Check sheet for the drawn part. Datum: minimum x, y, z corner. Units: mm. A direction names the side the tool comes from. Round coordinates to 2 decimals unless told otherwise and drop trailing zeros. Order: outer loops, then holes, each group sorted by start corner. A loop starts at its lowest first (then second) coordinate and runs counter-clockwise, first axis right, second up. Notation, with made-up numbers: (56.25, 75.5) -> (100.25, 75.5) arc R20 ccw to (100.25, 92.5) -> close; hole circle Ø6 at (-39, -23). An arc over 180 degrees is marked (long way). Use CSV: the item, a comma, the result in double quotes.
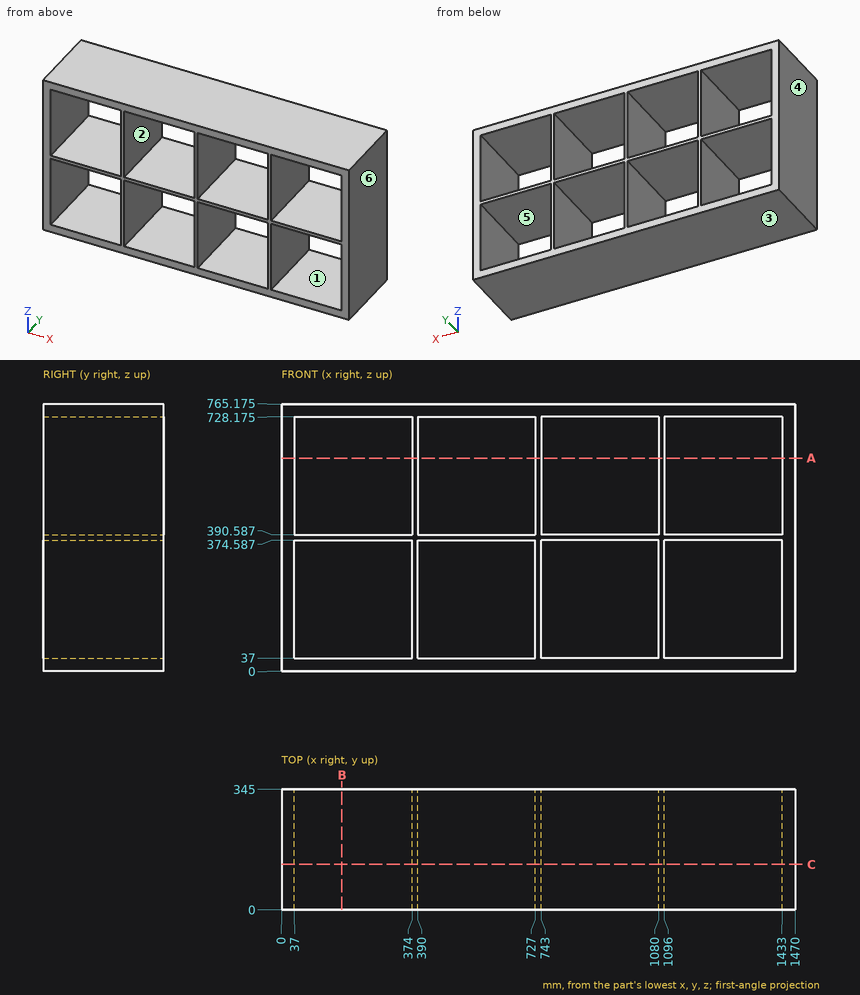
Q1. Sectioned sample at C-C, the plane y = 130. State how many separate pieces and enclosed holes the cut face has, then the cut area to 3 significant figures.
Result sheet:
separate pieces,"1"
enclosed holes,"8"
area,"215,000 mm^2"
Q2. Mould release check, pull along X, two halves, no side actions. Record for the marked faces 1, 2, 3 and 4: pulls with the +X half, pulls with the -X half, needs draft (parallel to the pull), parting line crosses it, or undercut.
Result sheet:
face 1,"undercut"
face 2,"undercut"
face 3,"needs draft"
face 4,"pulls with the -X half"
Q3. Sectioned sample at B-B, the plane x = 173. Enter the section's corners in (y, z) (1 decimal), then the cut area to 4 significant figures.
Result sheet:
outline,"(0, 0) -> (345, 0) -> (345, 37) -> (0, 37) -> close; (0, 374.6) -> (345, 374.6) -> (345, 390.6) -> (0, 390.6) -> close; (0, 728.2) -> (345, 728.2) -> (345, 765.2) -> (0, 765.2) -> close"
area,"31,050 mm^2"
Q4. Sectioned sample at A-A, the plane z = 610.5. Enter the section's corners in (x, y).
Result sheet:
outline,"(0, 0) -> (37, 0) -> (37, 345) -> (0, 345) -> close; (374, 0) -> (390, 0) -> (390, 345) -> (374, 345) -> close; (727, 0) -> (743, 0) -> (743, 345) -> (727, 345) -> close; (1080, 0) -> (1096, 0) -> (1096, 345) -> (1080, 345) -> close; (1433, 0) -> (1470, 0) -> (1470, 345) -> (1433, 345) -> close"
Q5. Access from +Z, -Z, +X, -X, +Y, -Y to the whole of each face (thin tool, end or side, straight path). Record for the marked faces 5 and 6.
Result sheet:
face 5,"+Y, -Y"
face 6,"+Z, -Z, +X, +Y, -Y"
Q6. Scan lines: L1, parallel to X at y = 96.5, z = 89; L2, parallel to Z at x = 256, y = 83 (1 decimal). Record each from-to range of solid material in increasing order.
Result sheet:
L1,"x = 0 to 37, 374 to 390, 727 to 743, 1080 to 1096, 1433 to 1470"
L2,"z = 0 to 37, 374.6 to 390.6, 728.2 to 765.2"
